Can you work these out from the model? Positions are in its coordinate system, mm. Round coordinates to 2 decimals unless told otherwise and drop trailing zeros. Loops run counter-clockwise (first coordinate to the right, second up) from the corner with the lowest first, then second, coordinate; pieces in that order, holes last. Notation, with made-up numbers: (29, -11) -> (78, -11) arc R20 ccw to (78, 18) -> close; hole circle Ø2 at (27.25, 43.5). An arc over 180 degrees is marked (long way). Answer as a JSON object with one key per item and string values.
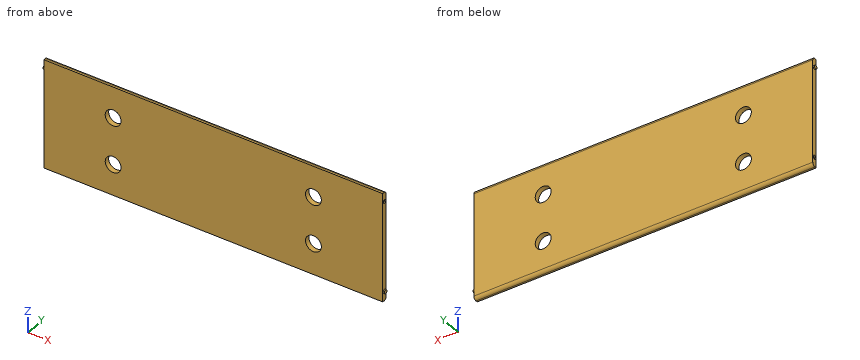
```python
from build123d import *

# Parameters (mm, degrees)
BOSS_EXTRUDE1_DEPTH            = 22.225
CUT_EXTRUDE1_REACH             = 331.298
SKETCH2_R                      = 4.7625
CUT_EXTRUDE1_DIRECTION_2_REACH = 331.298
CUT_EXTRUDE2_DEPTH             = 254
FILLET1_R                      = 12.7
FILLET4_R                      = 1.2446
F_1_4_CLEARANCE_HOLE1_D        = 6.5278
F_1_4_CLEARANCE_HOLE1_DEPTH    = 6.35
F_1_4_CLEARANCE_HOLE1_TIP      = 1.961148974
SKETCH6_W                      = 65.609477097
SKETCH6_H                      = 246.187780251
CUT_EXTRUDE3_DEPTH             = 200.66
SKETCH7_W                      = 53.894876093
SKETCH7_H                      = 277.088175353
CUT_EXTRUDE4_DEPTH             = 200.66
SKETCH8_R                      = 0.762
BOSS_EXTRUDE2_DEPTH            = 0.508
SKETCH9_R                      = 0.762
CUT_EXTRUDE5_DEPTH             = 0.508
SKETCH10_R                     = 0.762
CUT_EXTRUDE6_DEPTH             = 0.508
SKETCH11_R                     = 0.762
BOSS_EXTRUDE3_DEPTH            = 0.508


with BuildPart() as part:
    # Sketch1 → Boss-Extrude1 (new, symmetric)
    with BuildSketch(Plane.XY):
        with BuildLine():
            add(Edge.make_bspline(
                [(245.618, 12.7), (245.618, 14.831688899), (245.575395866, 19.120958406), (245.322441099, 27.489835839), (244.696729955, 37.702743517), (243.466672055, 49.517673174), (241.209008074, 64.702111997), (237.26896978, 82.613605898), (230.879834274, 102.41559311), (222.956422719, 120.542434531), (213.624406237, 137.012147223), (203.008125467, 151.842675097), (187.304904565, 169.454437631), (165.078062417, 187.457160851), (135.224023579, 202.760511588), (108.503296863, 210.348405687), (86.529134162, 213.367524052), (75.40386678, 213.868), (69.85, 213.868)],
                knots=[0, 0, 0, 0, 0.015625, 0.03125, 0.0625, 0.09375, 0.125, 0.1875, 0.25, 0.3125, 0.375, 0.4375, 0.5, 0.625, 0.75, 0.875, 0.9375, 1, 1, 1, 1], degree=3))
            Line((69.85, 213.868), (-69.85, 213.868))
            add(Edge.make_bspline(
                [(-69.85, 213.868), (-75.40386678, 213.868), (-86.529134162, 213.367524052), (-108.503296863, 210.348405687), (-135.224023579, 202.760511588), (-165.078062417, 187.457160851), (-187.304904565, 169.454437631), (-203.008125467, 151.842675097), (-213.624406237, 137.012147223), (-222.956422719, 120.542434531), (-230.879834274, 102.41559311), (-237.26896978, 82.613605898), (-241.209008074, 64.702111997), (-243.466672055, 49.517673174), (-244.696729955, 37.702743517), (-245.322441099, 27.489835839), (-245.575395866, 19.120958406), (-245.618, 14.831688899), (-245.618, 12.7)],
                knots=[0, 0, 0, 0, 0.0625, 0.125, 0.25, 0.375, 0.5, 0.5625, 0.625, 0.6875, 0.75, 0.8125, 0.875, 0.90625, 0.9375, 0.96875, 0.984375, 1, 1, 1, 1], degree=3))
            Line((-245.618, 12.7), (-245.618, -12.7))
            Line((-245.618, -12.7), (-247.65, -12.7))
            Line((-247.65, -12.7), (-247.65, 12.7))
            add(Edge.make_bspline(
                [(-69.85, 215.9), (-159.851901214, 215.9), (-247.65, 151.138652105), (-247.65, 12.7)],
                knots=[0, 0, 0, 0, 1, 1, 1, 1], degree=3))
            Line((-69.85, 215.9), (69.85, 215.9))
            add(Edge.make_bspline(
                [(247.65, 12.7), (247.65, 151.138652105), (159.851901214, 215.9), (69.85, 215.9)],
                knots=[0, 0, 0, 0, 1, 1, 1, 1], degree=3))
            Line((247.65, 12.7), (247.65, -12.7))
            Line((247.65, -12.7), (245.618, -12.7))
            Line((245.618, -12.7), (245.618, 12.7))
        make_face()
    extrude(amount=BOSS_EXTRUDE1_DEPTH, both=True)

    # Sketch2 → Cut-Extrude1 (cut, up to next)
    with BuildSketch(Plane(origin=(0, 0, 0), x_dir=(0, 0, -1), z_dir=(1, 0, 0)), mode=Mode.PRIVATE) as cut_extrude1_sk1:
        with Locations(Location((0, 0, 0), (0, 0, 180))):
            Circle(SKETCH2_R)
    cut_extrude1_tool1 = extrude(cut_extrude1_sk1.sketch, amount=-CUT_EXTRUDE1_REACH, mode=Mode.PRIVATE) & part.part
    add(cut_extrude1_tool1.solids().sort_by_distance((0, 0, 0))[0], mode=Mode.SUBTRACT)

    # Sketch2 → Cut-Extrude1 direction 2 (cut, up to next)
    with BuildSketch(Plane(origin=(0, 0, 0), x_dir=(0, 0, -1), z_dir=(1, 0, 0)), mode=Mode.PRIVATE) as cut_extrude1_direction_2_sk1:
        with Locations(Location((0, 0, 0), (0, 0, 180))):
            Circle(SKETCH2_R)
    cut_extrude1_direction_2_tool1 = extrude(cut_extrude1_direction_2_sk1.sketch, amount=CUT_EXTRUDE1_DIRECTION_2_REACH, mode=Mode.PRIVATE) & part.part
    add(cut_extrude1_direction_2_tool1.solids().sort_by_distance((0, 0, 0))[0], mode=Mode.SUBTRACT)

    # Sketch3 → Cut-Extrude2 (cut, symmetric)
    with BuildSketch(Plane(origin=(0, 0, 0), x_dir=(0, 0, -1), z_dir=(1, 0, 0))):
        Polygon((-22.225, 215.9), (-12.7, -12.7), (-47.625, -12.7), (-47.625, 215.9), align=None)
        Polygon((22.225, 215.9), (12.7, -12.7), (47.625, -12.7), (47.625, 215.9), align=None)
    extrude(amount=CUT_EXTRUDE2_DEPTH, both=True, mode=Mode.SUBTRACT)

    # Fillet1
    fillet1_edges = [part.edges().sort_by_distance(p)[0] for p in [
        (-246.634, -12.7, 12.7),
        (246.634, -12.7, 12.7),
        (-246.634, -12.7, -12.7),
        (246.634, -12.7, -12.7),
    ]]
    fillet(fillet1_edges, radius=FILLET1_R)

    # Fillet4
    fillet4_edges = [part.edges().sort_by_distance(p)[0] for p in [
        (-247.65, 6.085646041, 13.482735252),
        (-247.65, -9.165276607, 9.309489742),
        (-247.65, -9.165276607, -9.309489742),
        (247.65, 6.085646041, 13.482735252),
        (247.65, -12.7, 0),
        (247.65, -9.165276607, 9.309489742),
        (247.65, -9.165276607, -9.309489742),
        (0, 215.9, -22.225),
        (0, 215.9, 22.225),
        (-203.084938623, 154.469294773, 19.665387282),
        (203.084938625, 154.469294774, 19.665387282),
        (247.65, 6.085646041, -13.482735252),
        (203.084938625, 154.469294774, -19.665387282),
        (-203.084938623, 154.469294773, -19.665387282),
        (-247.65, 6.085646041, -13.482735252),
        (-247.65, -12.7, 0),
    ]]
    fillet(fillet4_edges, radius=FILLET4_R)

    # 1_4 Clearance Hole1
    with Locations(Plane(origin=(5.734151724, 215.9, -6.658847299), x_dir=(1, 0, 0), z_dir=(0, 1, 0))):
        with Locations((35.540848276, -16.183847299), (35.540848276, 2.866152701), (-47.009151724, -16.183847299), (-47.009151724, 2.866152701)):
            Hole(F_1_4_CLEARANCE_HOLE1_D / 2, depth=F_1_4_CLEARANCE_HOLE1_DEPTH)
            with Locations((0, 0, -(F_1_4_CLEARANCE_HOLE1_DEPTH + F_1_4_CLEARANCE_HOLE1_TIP / 2))):  # 118° drill point
                Cone(0, F_1_4_CLEARANCE_HOLE1_D / 2, F_1_4_CLEARANCE_HOLE1_TIP, mode=Mode.SUBTRACT)

    # Sketch6 → Cut-Extrude3 (cut)
    with BuildSketch(Plane.ZY.offset(-69.85)):
        with Locations((-2.573891908, 99.039872329)):
            Rectangle(SKETCH6_W, SKETCH6_H)
    extrude(amount=-CUT_EXTRUDE3_DEPTH, mode=Mode.SUBTRACT)

    # Sketch7 → Cut-Extrude4 (cut)
    with BuildSketch(Plane.ZY.offset(69.85)):
        with Locations((-0.531372719, 92.342266691)):
            Rectangle(SKETCH7_W, SKETCH7_H)
    extrude(amount=CUT_EXTRUDE4_DEPTH, mode=Mode.SUBTRACT)

    # Sketch8 → Boss-Extrude2 (add)
    with BuildSketch(Plane(origin=(69.85, 0, 0), x_dir=(0, 0, -1), z_dir=(1, 0, 0))):
        with Locations(Location((18.330333333, 214.884, 0), (0, 0, 90))):
            Circle(SKETCH8_R)
    extrude(amount=BOSS_EXTRUDE2_DEPTH)

    # Sketch9 → Cut-Extrude5 (cut)
    with BuildSketch(Plane(origin=(69.85, 0, 0), x_dir=(0, 0, -1), z_dir=(1, 0, 0))):
        with Locations(Location((-18.330333333, 214.884, 0), (0, 0, 90))):
            Circle(SKETCH9_R)
    extrude(amount=-CUT_EXTRUDE5_DEPTH, mode=Mode.SUBTRACT)

    # Sketch10 → Cut-Extrude6 (cut)
    with BuildSketch(Plane.ZY.offset(69.85)):
        with Locations(Location((-18.330333333, 214.884, 0), (0, 0, 90))):
            Circle(SKETCH10_R)
    extrude(amount=-CUT_EXTRUDE6_DEPTH, mode=Mode.SUBTRACT)

    # Sketch11 → Boss-Extrude3 (add)
    with BuildSketch(Plane.ZY.offset(69.85)):
        with Locations(Location((18.330333333, 214.884, 0), (0, 0, 90))):
            Circle(SKETCH11_R)
    extrude(amount=BOSS_EXTRUDE3_DEPTH)


solid = part.part
```
Q1. I want a section at A-A, the plane z = -8. Write out the boundary of the cut face in (x, y), then the cut area to 3 significant figures.
Determined:
{"outline": "(-69.85, 213.87) -> (-44.16, 213.87) -> (-44.16, 215.9) -> (-69.85, 215.9) -> close; (-38.39, 213.87) -> (38.39, 213.87) -> (38.39, 215.9) -> (-38.39, 215.9) -> close; (44.16, 213.87) -> (69.85, 213.87) -> (69.85, 215.9) -> (44.16, 215.9) -> close", "area": "260 mm²"}
Q2. If I drill on L1, parallel to X at y = 214.2, z = -11.5; L2, parallel to X at y = 215.3, z = 12.5; L3, parallel to Z at x = 63, y = 214.25, over which ranges is the centre line in solid material (lowest first)? Write a range as [from, to].
Determined:
{"L1": "[-69.85, -43.87], [-38.68, 38.68], [43.87, 69.85]", "L2": "[-69.85, -42.62], [-39.93, 39.93], [42.62, 69.85]", "L3": "[-22.16, 22.16]"}
Q3. I want a section at B-B, the plane y = 215.15. Write out the boundary of the cut face in (x, z) (3 decimals).
Determined:
{"outline": "(-70.358, 17.616) -> (-69.85, 17.616) -> (-69.85, -17.616) -> (-69.342, -17.616) -> (-69.342, -19.044) -> (-69.85, -19.044) -> (-69.85, -22.07) -> (69.85, -22.07) -> (69.85, -19.044) -> (70.358, -19.044) -> (70.358, -17.616) -> (69.85, -17.616) -> (69.85, 17.616) -> (69.342, 17.616) -> (69.342, 19.044) -> (69.85, 19.044) -> (69.85, 22.07) -> (-69.85, 22.07) -> (-69.85, 19.044) -> (-70.358, 19.044) -> close; hole circle Ø6.528 at (-41.275, -9.525); hole circle Ø6.528 at (-41.275, 9.525); hole circle Ø6.528 at (41.275, -9.525); hole circle Ø6.528 at (41.275, 9.525)"}
Q4. I want a section at C-C, the plane x = 40. Write out the boundary of the cut face in (y, z), then the cut area to 3 significant figures.
Determined:
{"outline": "(213.87, -22.14) -> (214.6, -22.17) arc R1.24 ccw to (215.9, -20.93) -> (215.9, -12.53) -> (213.87, -12.53) -> close; (213.87, -6.52) -> (215.9, -6.52) -> (215.9, 6.52) -> (213.87, 6.52) -> close; (213.87, 12.53) -> (215.9, 12.53) -> (215.9, 20.93) arc R1.24 ccw to (214.6, 22.17) -> (213.87, 22.14) -> close", "area": "65.0 mm²"}
Q5. I'm going to push flat-ended pins straight in: pin 1 (5 mm diameter, centred on x = 41.275, z = -9.525, fed in from +Y); pin 2 (1.2 mm diameter, centred on y = 214.5, z = 18.5, fed in from +X); pin 3 (1 mm diameter, centred on y = 215, z = 2.5, fed in from -X); pin 4 (0.9 mm diameter, centred on y = 214.88, z = -18.33, fed in from -X). Where does each tip first touch, or does it pass through?
Determined:
{"pin 1": "through", "pin 2": "x = 69.85", "pin 3": "x = -69.85", "pin 4": "x = -69.34"}
